from build123d import *

# Parameters (mm, degrees)
EXTRUDE_1_DEPTH     = 51
SKETCH_2_R          = 2.25
CUT_EXTRUDE_1_DEPTH = 56.456379254
FILLET_1_R          = 9


with BuildPart() as part:
    # Эскиз1 → Бобышка-Вытянуть1 (new body)
    with BuildSketch(Plane(origin=(0, 0, 0), x_dir=(1, 0, 0), z_dir=(0, 1, 0))):
        Polygon((0, 0), (10.6, 0), (10.6, 9.097791798), (15.1, 9.097791798), (15.1, -5), (-4.5, -5), (-4.5, 9.5), (0, 9.5), align=None)
    extrude(amount=EXTRUDE_1_DEPTH)

    # Эскиз2 → Вырез-Вытянуть1 (cut, through all)
    with BuildSketch(Plane(origin=(15.1, 0, 0), x_dir=(0, 0, -1), z_dir=(1, 0, 0))):
        with Locations((4.597791798, 42)):
            Circle(SKETCH_2_R)
        with Locations((4.597791798, 16)):
            Circle(SKETCH_2_R)
    extrude(amount=-CUT_EXTRUDE_1_DEPTH, mode=Mode.SUBTRACT)

    # Скругление1
    fillet_1_edges = [part.edges().sort_by_distance(p)[0] for p in [
        (12.85, 51, -9.097791798),
        (-2.25, 51, -9.5),
    ]]
    fillet(fillet_1_edges, radius=FILLET_1_R)


solid = part.part
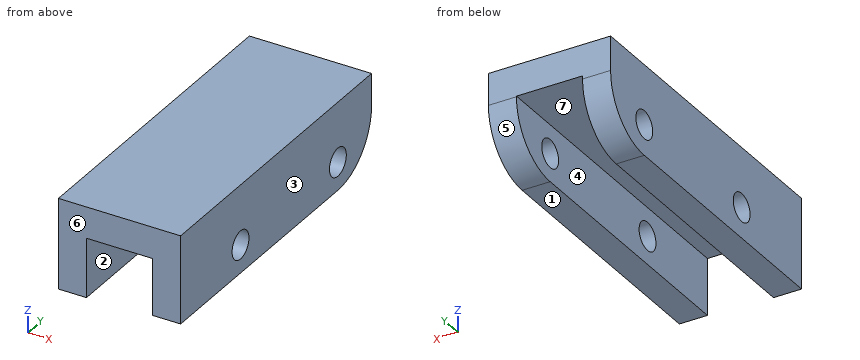
For this review, take the finished solid that the model builds, in its own axes (mm). Face numbers are marked on the shaded views. A direction names the side the tool comes from. Round coordinates to 2 decimals unless told otherwise and drop trailing zeros. Order: outer loops, then holes, each group sorted by start corner. A loop starts at its lowest first (then second) coordinate and runs counter-clockwise, first axis right, second up. Notation, with made-up numbers: M 5,88 L 21,88 A18 ccw 21,122 Z; hole C 17,-21.75 d6. An arc over 180 degrees is marked long. Write each question's results on one line, items separated by ' | '. Start each with the question number.
1. Add section D-D (z = -4.5). State the section outline as (x, y) points, then the cut area to 3 significant figures.
2. Draft analysis for pull direction X (two halves, no side actions). For the marked faces 1, 2, 3 and 4, state which applies: pulls with the +X half, pulls with the -X half, needs draft (parallel to the pull), parting line crosses it, or undercut.
3. Add section B-B (x = 13). State the section outline as (y, z) points, then the cut area to 3 significant figures.
4. Clearance check with flat-ended pins moving along their axes: pin 1 Ø1 at (x, z) = (-1.5, -7) entering from +Y; pin 2 Ø4 at (x, z) = (6, -3.5) entering from +Y; pin 3 Ø3.5 at (x, y) = (14, 23.5) entering from -Z; pin 4 Ø5 at (x, z) = (0, -7.5) entering from +Y. State where each tip first meets the part, or that it passes through.
5. To check wall thickness, follow L1, parallel to X at y = 30.5, z = -5; L2, parallel to Y at x = -0.5, z = -5.75; L3, parallel to Y at x = -0.5, z = -5.5. State the ranges of each line that lie inside material, in increasing order. Write a range as [from, to].
6. Tool access review of the marked faces 5, 6 and 7: name each direction out of +Z, -Z, +X, -X, +Y, -Y from which nothing blocks a thin tool from reaching the whole face with its end or side.
7. Add section C-C (z = -1.5). State the section outline as (x, y) points, then the cut area to 3 significant figures.
8. Add section A-A (y = 16). State the section outline as (x, z) points, then the cut area to 3 significant figures.
Output values:
1) outline: M -4.5,0 L 0,0 L 0,13.75 L -4.5,13.75 Z; M -4.5,18.25 L 0,18.25 L 0,39.75 L -4.5,39.75 Z; M -4.5,44.25 L 0,44.25 L 0,50.06 L -4.5,50.06 Z; M 10.6,0 L 15.1,0 L 15.1,13.75 L 10.6,13.75 Z; M 10.6,18.25 L 15.1,18.25 L 15.1,39.75 L 10.6,39.75 Z; M 10.6,44.25 L 15.1,44.25 L 15.1,49.85 L 10.6,49.85 Z | area: 369 mm^2
2) face 1: needs draft | face 2: undercut | face 3: pulls with the +X half | face 4: undercut
3) outline: M 0,-9.1 L 42,-9.1 A9 ccw 51,-0.1 L 51,5 L 0,5 Z; hole C 16,-4.6 d4.5; hole C 42,-4.6 d4.5 | area: 670 mm^2
4) pin 1: y = 48.71 | pin 2: through | pin 3: z = -9.1 | pin 4: y = 49.79
5) L1: [-4.5, 0], [10.6, 15.1] | L2: [0, 14.07], [17.93, 40.07], [43.93, 49.31] | L3: [0, 13.94], [18.06, 39.94], [44.06, 49.48]
6) face 5: -Z, +X, +Y | face 6: +Z, -Z, +X, -X, -Y | face 7: -Z, +Y, -Y
7) outline: M -4.5,0 L 0,0 L 0,50.94 L -4.5,50.94 Z; M 10.6,0 L 15.1,0 L 15.1,50.89 L 10.6,50.89 Z | area: 458 mm^2
8) outline: M -4.5,-9.5 L 0,-9.5 L 0,-6.85 L -4.5,-6.85 Z; M -4.5,-2.35 L 0,-2.35 L 0,0 L 10.6,0 L 10.6,-2.35 L 15.1,-2.35 L 15.1,5 L -4.5,5 Z; M 10.6,-9.1 L 15.1,-9.1 L 15.1,-6.85 L 10.6,-6.85 Z | area: 141 mm^2
